```python
from build123d import *

# Parameters (mm, degrees)
F0_W     = 50
F0_H     = 20.75
F3_DEPTH = 50.001
F4_COUNT = 9


with BuildPart() as f1:
    # F0 (on Front) → F1 (revolve)
    with BuildSketch(Plane.XZ):
        with Locations((-25, 19.875)):
            Rectangle(F0_W, F0_H)
    revolve(axis=Axis((-20.0732499361, 0, 0), (1, 0, 0)))

    # F2 (on face) → F3 (cut, through all)
    with BuildSketch(Plane.YZ):
        with BuildLine():
            ThreePointArc((-8.6240252272, 15.9361409658), (-6.1974049971, 17.0272302886), (-3.6371673564, 17.7512087932))
            ThreePointArc((-3.6371673564, 17.7512087932), (-3.4777696522, 23.9342534629), (-3, 30.1008720804))
            ThreePointArc((-3, 30.1008720804), (-10.3461093356, 28.4257017788), (-17.0503342847, 24.9869686193))
            ThreePointArc((-17.0503342847, 24.9869686193), (-12.7205154565, 20.5701691072), (-8.6240252272, 15.9361409658))
        make_face()
    f3 = extrude(amount=-F3_DEPTH, mode=Mode.SUBTRACT)

    # F4: F3 ×9 about axis
    f4_axis = Axis((-20.0732499361, 0, 0), (1, 0, 0))
    for i in range(1, F4_COUNT):
        add(f3.rotate(f4_axis, i * 360 / F4_COUNT), mode=Mode.SUBTRACT)


solid = f1.part
```
Geometry check sheet. Reference: the model listing, model coordinates, mm. A direction names the side the tool comes from. Round coordinates to 2 decimals unless told otherwise and drop trailing zeros. Order: outer loops, then holes, each group sorted by start corner. A loop starts at its lowest first (then second) coordinate and runs counter-clockwise, first axis right, second up. Notation, with made-up numbers: M 29,68.5 L 47,68.5 A27 ccw 47,88.5 Z; hole C -31.75,51.25 d1. An arc over 180 degrees is marked long. Write item = value, one per line.
Q1. Section check C-C (z = 13.5). Enter the section's corners in (x, y), plus the area to 3 significant figures.
Answer block:
outline = M -50,-16.03 L 0,-16.03 L 0,16.03 L -50,16.03 Z
area = 1,600 mm^2
Q2. Scan lines: line 1 (Z direction, x = -44, y = 0.5); line 2 (Z direction, x = -7.5, y = -19.5); line 3 (Y direction, x = -40.5, z = -6.5). Record each from-to range of solid material in increasing order.
Answer block:
line_1 = -18.11 to -9.49, 9.49 to 30.25
line_2 = -15.24 to -7.09, -0.25 to 7.1, 18.06 to 23.13
line_3 = -18.51 to -6.93, 6.93 to 18.51
Q3. Release check for a two-part mould opening along Z. For faces 4 (the cylindrical face through (-24.65, -18.91, -14.94)), 5 (the flat face through (0, 6, 8)), 6 (the cylindrical face through (-24.65, -22.539, -9.002)) record: released by +Z, released by -Z, zero draft, split by the parting line, or undercut.
Answer block:
face_4 = released by -Z
face_5 = zero draft
face_6 = undercut
Q4. Depth check by flat-ended pin: pin 1 Ø8 at (x, z) = (-44.5, -13.5) entering from -Y; pin 2 Ø1 at (x, y) = (-16.5, -15.5) entering from -Z; pin 3 Ø12 at (x, y) = (-30.5, -13.5) entering from -Z. Enter the tip coordinate at first touch or a pass-through.
Answer block:
pin_1 = -27.57
pin_2 = -13.4
pin_3 = -29.31
Q5. Section check B-B (y = -19.5). Enter the section's corners in (x, z).
Answer block:
outline = M -50,-15.24 L 0,-15.24 L 0,-7.09 L -50,-7.09 Z; M -50,-0.25 L 0,-0.25 L 0,7.1 L -50,7.1 Z; M -50,18.06 L 0,18.06 L 0,23.13 L -50,23.13 Z
Q6. Section check A-A (y = 0). Enter the section's corners in (x, z).
Answer block:
outline = M -50,-18.12 L 0,-18.12 L 0,-9.5 L -50,-9.5 Z; M -50,9.5 L 0,9.5 L 0,30.25 L -50,30.25 Z
Q7. Set-up check for faces 1 (the cylindrical face through (-24.65, -4.884, -23.601)), 2 (the cylindrical face through (-24.65, 6.16, 17.04)), 3 (the cylindrical face through (-24.65, 15.674, 9.092)): record each of +Z, -Z, +X, -X, +Y, -Y from which the full face is reachable in a straight line by a thin tool's end or side.
Answer block:
face_1 = -Z, +X, -X
face_2 = +Z, +X, -X
face_3 = +X, -X
